```python
from build123d import *

# Parameters (mm, degrees)
F1_DEPTH = 25.4


with BuildPart() as f1:
    # F0 (on Top) → F1 (new body, symmetric)
    with BuildSketch(Plane.XY):
        with BuildLine():
            Line((21.971458, 0), (10.902476, 0))
            ThreePointArc((10.902476, 0), (7.811772, -7.605275), (0.292004, -10.898565))
            Line((0.292004, -10.898565), (0.292004, -21.608541))
            Line((0.292004, -21.608541), (2.044055, -21.608541))
            ThreePointArc((2.044055, -21.608541), (16.229103, -14.697197), (21.971458, 0))
        make_face()
        with BuildLine():
            ThreePointArc((0.292004, -10.898565), (-7.811772, 7.605275), (10.902476, 0))
            Line((10.902476, 0), (21.971458, 0))
            ThreePointArc((21.971458, 0), (-15.645094, 14.697197), (2.044055, -21.608541))
            Line((2.044055, -21.608541), (0.292004, -21.608541))
            Line((0.292004, -21.608541), (0.292004, -10.898565))
        make_face()
        with BuildLine():
            Line((116.802923, 0), (21.971458, 0))
            ThreePointArc((21.971458, 0), (16.229103, -14.697197), (2.044055, -21.608541))
            Line((2.044055, -21.608541), (116.802923, -21.608541))
            Line((116.802923, -21.608541), (116.802923, 0))
        make_face()
    extrude(amount=F1_DEPTH, both=True)


solid = f1.part
```
Verification items for the finished model (mm, model axes). A direction names the side the tool comes from. Coordinates: 2 decimals unless noted, no trailing zeros. Loops run counter-clockwise (first coordinate to the right, second up) from the corner with the lowest first, then second, coordinate; pieces in that order, holes last. Notation, with made-up numbers: (-30, 31.5) - (3, 31.5) arc R20 cw to (3, 67.5) - close; hole circle Ø3 at (-6.75, 18). An arc over 180 degrees is marked (long way). Return JSON: item names as keys, results as strings.
1. Section check A-A, the plane y = 3. Record the boundary of the cut face in (x, z).
Established:
{"outline": "(-21.18, -25.4) - (-10.48, -25.4) - (-10.48, 25.4) - (-21.18, 25.4) - close; (10.48, -25.4) - (21.76, -25.4) - (21.76, 25.4) - (10.48, 25.4) - close"}
2. Section check D-D, the plane x = 71. Record the boundary of the cut face in (y, z), then the cut area to 3 significant figures.
Established:
{"outline": "(-21.61, -25.4) - (0, -25.4) - (0, 25.4) - (-21.61, 25.4) - close", "area": "1,100 mm2"}
3. Section check C-C, the plane z = -1. Record the boundary of the cut face in (x, y), then the cut area to 3 significant figures.
Established:
{"outline": "(2.04, -21.61) - (116.8, -21.61) - (116.8, 0) - (21.97, 0) arc R21.68 ccw (long way) to start; hole circle Ø21.8 at (0, 0)", "area": "3,250 mm2"}
4. Tool access check on faces 1 (the flat face through (47, -5, -25.4)), 2 (the flat face through (70, 0, 0)). Record the directions out of +Z, -Z, +X, -X, +Y, -Y that give a thin tool (end or side, any length) a straight path to the whole face; none if there is none.
Established:
{"face 1": "-Z, +X, -X, +Y, -Y", "face 2": "+Z, -Z, +X, +Y"}
5. Go/stop test with flat-tipped pins: pin 1 (3 mm diameter, centred on x = 69.5, z = 6, fed in from -Y); pin 2 (15 mm diameter, centred on x = 54, z = -11, fed in from +Y). Record where each tip stops, or that it passes through.
Established:
{"pin 1": "stops at y = -21.61", "pin 2": "stops at y = 0"}
6. Thickness scan on L1, parallel to Y at x = 0, z = 1; L2, parallel to X at y = -2, z = -19 (3 decimals); L3, parallel to Y at x = 56, z = -2.5. Record the ranges inside material, lowest first.
Established:
{"L1": "y = -21.68 to -10.9, 10.9 to 21.68", "L2": "x = -21.295 to -10.717, 10.717 to 116.803", "L3": "y = -21.61 to 0"}
7. Section check B-B, the plane x = -5. Record the boundary of the cut face in (y, z).
Established:
{"outline": "(-21.02, -25.4) - (-9.69, -25.4) - (-9.69, 25.4) - (-21.02, 25.4) - close; (9.69, -25.4) - (21.02, -25.4) - (21.02, 25.4) - (9.69, 25.4) - close"}
